Autodesk Inventor part; units mm, degrees
ref_plane "YZ Plane" through (0, 0, 0) normal (1, 0, 0) x (0, 1, 0)
ref_plane "XZ Plane" through (0, 0, 0) normal (0, 1, 0) x (-1, 0, 0)
ref_plane "XY Plane" through (0, 0, 0) normal (0, 0, 1) x (1, 0, 0)
sketch "main" plane through (0, 0, 0) normal (0, 0, 1) x (1, 0, 0)
  circle A0 centre (-198.1135, 49.9495) radius 2.1844
  circle A1 centre (-95.8324, -13.8772) radius 2.1
  arc A2 (-99.5351, -19.036) -> (-94.63, -7.6421) centre (-95.8324, -13.8772) ccw
  arc A3 (-204.4481, 49.5075) -> (-198.1135, 43.5995) centre (-198.1135, 49.9495) ccw
  line L0 (-210.7981, 140.5057) -> (-204.4481, 49.5075)
  arc A4 (-209.271, 140.8599) -> (-94.63, -7.6421) centre (115.0165, 272.7027) ccw
  circle A5 centre (-206.375, 125.4125) radius 2.0828
  line L1 (-198.1135, 43.5995) -> (-186.2072, 43.5995)
  arc A6 (-209.271, 140.8599) -> (-210.7981, 140.5057) centre (-210.0063, 140.561) ccw
  circle A7 centre (-135.2274, 18.1995) radius 2.0828
  line L2 (-185.4135, 15.8183) -> (-185.4135, 42.8058)
  line L3 (-198.1135, 15.0245) -> (-186.2072, 15.0245)
  arc A8 (-185.4135, 42.8058) -> (-186.2072, 43.5995) centre (-186.2072, 42.8058) ccw
  arc A9 (-186.2072, 15.0245) -> (-185.4135, 15.8183) centre (-186.2072, 15.8183) ccw
  line L4 (-199.4808, 2.4735) -> (-97.1997, -20.0783)
  circle A10 centre (-198.1135, 8.6745) radius 2.1848
  arc A11 (-198.1135, 15.0245) -> (-199.4808, 2.4735) centre (-198.1135, 8.6745) ccw
  point P0 (1.1251, 9.7944)
  point P1 (-211.1526, 145.5863)
  point P2 (-191.7635, 49.9495)
  dimension "d7" = 12.7
  dimension "d8" = 4.1656
  dimension "d9" = 6.35
  dimension "d11" = 0.7937
  dimension "d13" = 4.1656
  dimension "d16" = 0.7937
  dimension "d19" = 26.9875
  dimension "d20" = 0
  dimension "d21" = 6.35
  dimension "d24" = 6.35
sketch "Sketch1" plane through (0, 0, 0) normal (1, 0, 0) x (0, 1, 0)
  circle A0 centre (44.45, -15.875) radius 2.0955
  circle A1 centre (0, 0) radius 2.1844
  circle A2 centre (102.2811, -63.8268) radius 2.1
  arc A3 (98.5784, -68.9855) -> (103.4835, -57.5917) centre (102.2811, -63.8268) ccw
  arc A4 (-6.3346, -0.442) -> (0, -6.35) centre (0, 0) ccw
  line L0 (-12.6846, 90.5562) -> (-6.3346, -0.442)
  arc A5 (-11.1575, 90.9104) -> (103.4835, -57.5917) centre (313.1299, 222.7532) ccw
  circle A6 centre (-8.2615, 75.463) radius 2.0828
  line L1 (0, -6.35) -> (11.9063, -6.35)
  arc A7 (-11.1575, 90.9104) -> (-12.6846, 90.5562) centre (-11.8928, 90.6114) ccw
  circle A8 centre (62.8861, -31.75) radius 2.0828
  line L2 (12.7, -34.1313) -> (12.7, -7.1438)
  line L3 (0, -34.925) -> (11.9063, -34.925)
  arc A9 (12.7, -7.1438) -> (11.9063, -6.35) centre (11.9063, -7.1437) ccw
  arc A10 (11.9063, -34.925) -> (12.7, -34.1313) centre (11.9063, -34.1313) ccw
  line L4 (-1.3673, -47.4761) -> (100.9138, -70.0278)
  circle A11 centre (0, -41.275) radius 2.1848
  arc A12 (0, -34.925) -> (-1.3673, -47.4761) centre (0, -41.275) ccw
  dimension "d18" = 4.191
extrude "Extrusion1" add sketch "Sketch1" along normal blind 1.5875
equation "\"BendRadius\" = Thickness"
equation "\"BendReliefWidth\" = Thickness"
equation "\"BendReliefDepth\" = 0.5 * Thickness"
equation "\"CornerReliefSize\" = 4 * Thickness"
equation "\"MinimumRemnant\" = 2 * Thickness"
equation "\"TransitionRadius\" = BendRadius"
equation "\"JacobiRadiusSize\" = BendRadius"
equation "\"GapSize\" = Thickness"
properties part number "Ramp V2" material "Acetal Resin, White"
Can you work these out from the model? Positions are in its coordinate system, mm. A direction names the side the tool comes from. Coordinates: 2 decimals unless noted, no trailing zeros. Loops run counter-clockwise (first coordinate to the right, second up) from the corner with the lowest first, then second, coordinate; pieces in that order, holes last. Notation, with made-up numbers: (29.5, 71) - (69.5, 71) arc R30 ccw to (69.5, 108) - close; hole circle Ø10 at (-11, 89.25). An arc over 180 degrees is marked (long way). Put each result on its own line as item: value. Start each with the question number.
Item 1: Suppose I cut it at B-B (z = -31.75). Please give me the cut outline in (x, y).
Item 2: Suppose I cut it at C-C (x = 1.1). State how many separate pieces and enclosed holes the cut face has, and give its area (3 significant figures).
Item 3: If I drill on line 1 along Z through (x, y) = (0.4, 44.45); line 2 along Z through (x, y) = (0.85, 101); line 3 along Z through (x, y) = (0.65, 0) (3 decimals), over which ranges is the centre line in solid material (lowest first)?
Item 4: Suppose I cut it at A-A (y = 44.45). Please give me the cut outline in (x, z), and give its area (3 significant figures).
Item 5: For pin 1 (0.8 mm diameter, centred on x = 0.5, z = -14.5, fed in from -Y), with a flat end and sliding along its axis, tell me the tip position at first contact or that it passes through.
Item 6: If we mould it in two halves opening along Y, with no side actions, what happens to faces 1 (the face through (0.78, 64.81, -30.95)), 2 (the face through (0.78, 36.84, 7.79)), 3 (the face through (0, 34, -19))? For each: +Y half, -Y half, draft (parallel to the pull), parting line (faces both ways), or undercut.
Item 7: Suppose I cut it at D-D (z = 32). Please give me the cut outline in (x, y).
Item 8: Which directions (+Z, -Z, +X, -X, +Y, -Y) give clear straight access to the entire face, cutting with the end or side of a thin tool? Please do faces 4 (the face through (0.78, -4.28, -4.69)), 5 (the face through (0.783, 49.057, -58.594)).
Here are the results:
1. outline: (0, 12.7) - (1.59, 12.7) - (1.59, 60.8) - (0, 60.8) - close; (0, 64.97) - (1.59, 64.97) - (1.59, 72.77) - (0, 72.77) - close
2. separate pieces: 1
2. enclosed holes: 6
2. area: 5,980 mm²
3. line 1: -57.58 to -17.97, -13.78 to -1.65
3. line 2: -70.05 to -65.49, -62.16 to -55.72
3. line 3: -47.778 to -43.46, -39.09 to -34.925, -6.35 to -2.184, 2.184 to 66.246
4. outline: (0, -57.58) - (1.59, -57.58) - (1.59, -17.97) - (0, -17.97) - close; (0, -13.78) - (1.59, -13.78) - (1.59, -1.65) - (0, -1.65) - close
4. area: 82.1 mm²
5. pin 1: y = 12.7
6. face 1: undercut
6. face 2: +Y half
6. face 3: draft
7. outline: (0, -8.6) - (1.59, -8.6) - (1.59, 19.6) - (0, 19.6) - close
8. face 4: +X, -X, -Y
8. face 5: -Z, +X, -X, -Y
